```python
from build123d import *

# Parameters (mm, degrees)
SKETCH1_R           = 2.5
SKETCH1_W           = 57
SKETCH1_H           = 22.5
BOSS_EXTRUDE1_DEPTH = 3
CUT_EXTRUDE1_DEPTH  = 83.677082677


with BuildPart() as part:
    # Sketch1 → Boss-Extrude1 (new body)
    # profile 1 of 8: a face of its own
    with BuildSketch(Plane.XY):
        with BuildLine():
            ThreePointArc((22.5, 0), (15.909902577, 15.909902577), (0, 22.5))
            Line((0, 22.5), (-22.5, 0))
            Line((-22.5, 0), (-22.124973736, -4.090909091))
            ThreePointArc((-22.124973736, -4.090909091), (2.054031517, -22.406047276), (22.5, 0))
        make_face()
        with BuildLine():
            ThreePointArc((-7.5, 5), (-9.267766953, 9.267766953), (-5, 7.5))
            Line((-5, 7.5), (-5, 9))
            Line((-5, 9), (-2.405779746, 18.179870439))
            ThreePointArc((-2.405779746, 18.179870439), (0, 20), (2.405779746, 18.179870439))
            Line((2.405779746, 18.179870439), (5, 9))
            Line((5, 9), (5, 7.5))
            ThreePointArc((5, 7.5), (7.5, 10), (10, 7.5))
            ThreePointArc((10, 7.5), (9.267766953, 5.732233047), (7.5, 5))
            Line((7.5, 5), (9, 5))
            Line((9, 5), (18.179870439, 2.405779746))
            ThreePointArc((18.179870439, 2.405779746), (19.493699588, 1.508363998), (20, 0))
            ThreePointArc((20, 0), (19.493699588, -1.508363998), (18.179870439, -2.405779746))
            Line((18.179870439, -2.405779746), (9, -5))
            Line((9, -5), (7.5, -5))
            ThreePointArc((7.5, -5), (9.267766953, -5.732233047), (10, -7.5))
            ThreePointArc((10, -7.5), (7.5, -10), (5, -7.5))
            Line((5, -7.5), (5, -9))
            Line((5, -9), (2.405779746, -18.179870439))
            ThreePointArc((2.405779746, -18.179870439), (0, -20), (-2.405779746, -18.179870439))
            Line((-2.405779746, -18.179870439), (-5, -9))
            Line((-5, -9), (-5, -7.5))
            ThreePointArc((-5, -7.5), (-9.267766953, -9.267766953), (-7.5, -5))
            Line((-7.5, -5), (-9, -5))
            Line((-9, -5), (-18.179870439, -2.405779746))
            ThreePointArc((-18.179870439, -2.405779746), (-20, 0), (-18.179870439, 2.405779746))
            Line((-18.179870439, 2.405779746), (-9, 5))
            Line((-9, 5), (-7.5, 5))
        make_face(mode=Mode.SUBTRACT)
    # profile 2 of 8: a face of its own
    with BuildSketch(Plane.XY):
        with Locations((-7.5, 7.5)):
            Circle(SKETCH1_R)
    # profile 3 of 8: a face of its own
    with BuildSketch(Plane.XY):
        with Locations((7.5, 7.5)):
            Circle(SKETCH1_R)
    # profile 4 of 8: a face of its own
    with BuildSketch(Plane.XY):
        with Locations((7.5, -7.5)):
            Circle(SKETCH1_R)
    # profile 5 of 8: a face of its own
    with BuildSketch(Plane.XY):
        with Locations((-7.5, -7.5)):
            Circle(SKETCH1_R)
    # profile 6 of 8: a face of its own
    with BuildSketch(Plane.XY):
        Polygon((-22.5, 22.5), (0, 22.5), (-22.5, 0), align=None)
    # profile 7 of 8: a face of its own
    with BuildSketch(Plane.XY):
        with Locations((-51, 11.25)):
            Rectangle(SKETCH1_W, SKETCH1_H)
    # profile 8 of 8: a face of its own
    with BuildSketch(Plane.XY):
        with BuildLine():
            Line((-22.5, 0), (-22.124973736, -4.090909091))
            ThreePointArc((-22.124973736, -4.090909091), (-23.843623821, -1.156469426), (-27.041634566, 0))
            Line((-27.041634566, 0), (-22.5, 0))
        make_face()
    extrude(amount=BOSS_EXTRUDE1_DEPTH)

    # Sketch4 → Cut-Extrude1 (cut, through all)
    with BuildSketch(Plane.XY.offset(3)):
        with BuildLine():
            Line((-79.5, 22.5), (0, 22.5))
            ThreePointArc((0, 22.5), (-17.295887583, 14.391048354), (-22.124973736, -4.090909091))
            ThreePointArc((-22.124973736, -4.090909091), (-23.843623821, -1.156469426), (-27.041634566, 0))
            Line((-27.041634566, 0), (-79.5, 0))
            Line((-79.5, 0), (-79.5, 22.5))
        make_face()
    extrude(amount=-CUT_EXTRUDE1_DEPTH, mode=Mode.SUBTRACT)


solid = part.part
```
Input: part model. Units: mm. Frame: model coordinates. Round coordinates to 2 decimals unless told otherwise and drop trailing zeros. Order: outer loops, then holes, each group sorted by start corner. A loop starts at its lowest first (then second) coordinate and runs counter-clockwise, first axis right, second up. Notation, with made-up numbers: (50, 11.25) - (81, 11.25) arc R28 ccw to (81, 37.25) - close; hole circle Ø11 at (1, 16). An arc over 180 degrees is marked (long way). One line per question, with ' | ' between items. Start each with the question number.
1) Pull-direction query (X, two-part tool) for faces 1 (the flat face through (-5, -8, 1)), 2 (the flat face through (-3.72, 13.53, 1.48)); classes: +X half, -X half, draft (parallel to the pull), parting line (faces both ways), or undercut.
2) Cut plane C-C, the plane x = 12.5. Return the cut outline in (y, z), then the cut area to 3 significant figures.
3) Contact query for flat-ended pins moving along their axis: P1, Ø3, axis at x = -15, y = 6.5, coming from the -Z side; P2, Ø1, axis at y = 13.5, z = 2.5, coming from the -X side; P3, Ø1.6, axis at y = -8, z = 1.5, coming from the +X side; P4, Ø1.5, axis at y = 11.5, z = 1, coming from the +X side. Output: stop coordinate, or through.
4) Cut plane B-B, the plane y = -17.5. Return the cut outline in (x, z).
5) Cut plane A-A, the plane z = 2.3. Return the cut outline in (x, y).
6) Ray query, probe 1 along X at (y, z) = (0, 1.35); probe 2 along Y at (x, z) = (-7, 2.4); probe 3 along Y at (x, z) = (1, 0.75). Return the intervals inside material, ascending.
Worked out:
1) face 1: undercut | face 2: undercut
2) outline: (-18.71, 0) - (-4.01, 0) - (-4.01, 3) - (-18.71, 3) - close; (4.01, 0) - (18.71, 0) - (18.71, 3) - (4.01, 3) - close | area: 88.2 mm^2
3) P1: stops at z = 0 | P2: stops at x = -18.36 | P3: stops at x = 21.32 | P4: stops at x = 19.77
4) outline: (-14.14, 0) - (-2.6, 0) - (-2.6, 3) - (-14.14, 3) - close; (2.6, 0) - (14.14, 0) - (14.14, 3) - (2.6, 3) - close
5) outline: circle Ø45 at (0, 0); hole (-18.18, -2.41) - (-9, -5) - (-7.5, -5) arc R2.5 cw to (-5, -7.5) - (-5, -9) - (-2.41, -18.18) arc R2.5 ccw to (2.41, -18.18) - (5, -9) - (5, -7.5) arc R2.5 cw to (7.5, -5) - (9, -5) - (18.18, -2.41) arc R2.5 ccw to (18.18, 2.41) - (9, 5) - (7.5, 5) arc R2.5 cw to (5, 7.5) - (5, 9) - (2.41, 18.18) arc R2.5 ccw to (-2.41, 18.18) - (-5, 9) - (-5, 7.5) arc R2.5 cw to (-7.5, 5) - (-9, 5) - (-18.18, 2.41) arc R2.5 ccw to start
6) probe 1: x = -22.5 to -20, 20 to 22.5 | probe 2: y = -21.38 to -5.05, 5.05 to 21.38 | probe 3: y = -22.48 to -19.79, 19.79 to 22.48
